```python
from build123d import *

# Parameters (mm, degrees)
BOSS_EXTRUDE1_DEPTH = 5.5
CUT_EXTRUDE1_DEPTH  = 3.5
SKETCH3_R           = 3
BOSS_EXTRUDE2_DEPTH = 3.5
SKETCH4_R           = 1.45
CUT_EXTRUDE2_DEPTH  = 5.5
SKETCH5_R           = 2.5
CUT_EXTRUDE3_DEPTH  = 2.6
CUT_EXTRUDE4_DEPTH  = 2
SKETCH7_W           = 3.5
SKETCH7_H           = 13.01
CUT_EXTRUDE5_DEPTH  = 1.55
SKETCH8_W           = 3.5
SKETCH8_H           = 12.6
CUT_EXTRUDE6_DEPTH  = 0.465


with BuildPart() as part:
    # Sketch1 → Boss-Extrude1 (new body)
    with BuildSketch(Plane.XY.offset(-5.5)):
        with BuildLine():
            Line((-30, -36), (30, -36))
            ThreePointArc((30, -36), (34.242640687, -34.242640687), (36, -30))
            Line((36, -30), (36, 30))
            ThreePointArc((36, 30), (34.242640687, 34.242640687), (30, 36))
            Line((30, 36), (-30, 36))
            ThreePointArc((-30, 36), (-34.242640687, 34.242640687), (-36, 30))
            Line((-36, 30), (-36, -30))
            ThreePointArc((-36, -30), (-34.242640687, -34.242640687), (-30, -36))
        make_face()
    extrude(amount=BOSS_EXTRUDE1_DEPTH)

    # Sketch2 → Cut-Extrude1 (cut)
    with BuildSketch(Plane.XY.offset(-3.5)):
        with BuildLine():
            Line((-30, -34), (30, -34))
            ThreePointArc((30, -34), (32.828427125, -32.828427125), (34, -30))
            Line((34, -30), (34, 30))
            ThreePointArc((34, 30), (32.828427125, 32.828427125), (30, 34))
            Line((30, 34), (-30, 34))
            ThreePointArc((-30, 34), (-32.828427125, 32.828427125), (-34, 30))
            Line((-34, 30), (-34, -30))
            ThreePointArc((-34, -30), (-32.828427125, -32.828427125), (-30, -34))
        make_face()
    extrude(amount=CUT_EXTRUDE1_DEPTH, mode=Mode.SUBTRACT)

    # Sketch3 → Boss-Extrude2 (add)
    with BuildSketch(Plane.XY.offset(-3.5)):
        with Locations((-30, 30)):
            Circle(SKETCH3_R)
        with Locations((30, 30)):
            Circle(SKETCH3_R)
        with Locations((-30, -30)):
            Circle(SKETCH3_R)
        with Locations((30, -30)):
            Circle(SKETCH3_R)
    extrude(amount=BOSS_EXTRUDE2_DEPTH)

    # Sketch4 → Cut-Extrude2 (cut)
    with BuildSketch(Plane.XY.offset(-5.5)):
        with Locations((-30, 30)):
            Circle(SKETCH4_R)
        with Locations((30, 30)):
            Circle(SKETCH4_R)
        with Locations((-30, -30)):
            Circle(SKETCH4_R)
        with Locations((30, -30)):
            Circle(SKETCH4_R)
    extrude(amount=CUT_EXTRUDE2_DEPTH, mode=Mode.SUBTRACT)

    # Sketch5 → Cut-Extrude3 (cut)
    with BuildSketch(Plane.XY.offset(-5.5)):
        with Locations((-30, 30)):
            Circle(SKETCH5_R)
        with Locations((30, 30)):
            Circle(SKETCH5_R)
        with Locations((-30, -30)):
            Circle(SKETCH5_R)
        with Locations((30, -30)):
            Circle(SKETCH5_R)
    extrude(amount=CUT_EXTRUDE3_DEPTH, mode=Mode.SUBTRACT)

    # Sketch6 → Cut-Extrude4 (cut)
    with BuildSketch(Plane.XY.offset(-5.5)):
        with BuildLine():
            Line((-16, -14), (-16, 14))
            ThreePointArc((-16, 14), (-15, 15), (-14, 14))
            Line((-14, 14), (-14, -14))
            ThreePointArc((-14, -14), (-15, -15), (-16, -14))
        make_face()
        with BuildLine():
            Line((-11, -14), (-11, 14))
            ThreePointArc((-11, 14), (-10, 15), (-9, 14))
            Line((-9, 14), (-9, -14))
            ThreePointArc((-9, -14), (-10, -15), (-11, -14))
        make_face()
        with BuildLine():
            Line((-6, -14), (-6, 14))
            ThreePointArc((-6, 14), (-5, 15), (-4, 14))
            Line((-4, 14), (-4, -14))
            ThreePointArc((-4, -14), (-5, -15), (-6, -14))
        make_face()
        with BuildLine():
            Line((-1, -14), (-1, 14))
            ThreePointArc((-1, 14), (0, 15), (1, 14))
            Line((1, 14), (1, -14))
            ThreePointArc((1, -14), (0, -15), (-1, -14))
        make_face()
        with BuildLine():
            Line((4, -14), (4, 14))
            ThreePointArc((4, 14), (5, 15), (6, 14))
            Line((6, 14), (6, -14))
            ThreePointArc((6, -14), (5, -15), (4, -14))
        make_face()
        with BuildLine():
            Line((9, -14), (9, 14))
            ThreePointArc((9, 14), (10, 15), (11, 14))
            Line((11, 14), (11, -14))
            ThreePointArc((11, -14), (10, -15), (9, -14))
        make_face()
        with BuildLine():
            Line((14, -14), (14, 14))
            ThreePointArc((14, 14), (15, 15), (16, 14))
            Line((16, 14), (16, -14))
            ThreePointArc((16, -14), (15, -15), (14, -14))
        make_face()
    extrude(amount=CUT_EXTRUDE4_DEPTH, mode=Mode.SUBTRACT)

    # Sketch7 → Cut-Extrude5 (cut)
    with BuildSketch(Plane.XY.offset(-1.55)):
        with Locations((35.25, -1.445)):
            Rectangle(SKETCH7_W, SKETCH7_H)
        with Locations((35.25, -20.495)):
            Rectangle(SKETCH7_W, SKETCH7_H)
    extrude(amount=CUT_EXTRUDE5_DEPTH, mode=Mode.SUBTRACT)

    # Sketch8 → Cut-Extrude6 (cut)
    with BuildSketch(Plane.XY.offset(-0.465)):
        with Locations((-35.25, -19)):
            Rectangle(SKETCH8_W, SKETCH8_H)
    extrude(amount=CUT_EXTRUDE6_DEPTH, mode=Mode.SUBTRACT)


solid = part.part
```
Read the model definition and answer for the solid it produces. Units are mm, in the model's axes. A direction names the side the tool comes from. Coordinates: 2 decimals unless noted, no trailing zeros. Write each loop counter-clockwise with the first axis right and the second up, starting at its lowest first coordinate (ties: lowest second). Pieces come first, ordered by that corner, then holes. Notation, with made-up numbers: (25, 65) -> (76, 65) arc R21 cw to (76, 92) -> close; hole circle Ø6 at (89, 24). An arc over 180 degrees is marked (long way). Answer as a JSON object with one key per item and string values.
Q1. A tool of negligible diameter and unlimited length cuts with its end or side. For faces 1 (the flat face through (-16, 0, -5)), 2 (the flat face through (32, -30, -2.9)), 3 (the cylindrical face through (27, 30, -2)), from which of +Z, -Z, +X, -X, +Y, -Y can it reach the whole face along a straight path? Write none if from no direction.
The answers:
{"face 1": "+Z, -Z", "face 2": "-Z", "face 3": "+Z"}
Q2. The part is cut by section C-C on z = -4.6. Give the number of separate pieces and of enclosed holes in the cut face, then the cut area to 3 significant figures.
The answers:
{"separate pieces": "1", "enclosed holes": "11", "area": "4,660 mm2"}
Q3. Determine the mould class of faces 4 (the cylindrical face through (-34.289, -34.196, -2.788)), 5 (the flat face through (35, -11, 0)), 6 (the flat face through (-6, 0, -5)) for opening direction Y: pulls with the +Y half, pulls with the -Y half, needs draft (parallel to the pull), parting line crosses it, or undercut.
The answers:
{"face 4": "pulls with the -Y half", "face 5": "needs draft", "face 6": "undercut"}
Q4. The part is cut by section B-B on y = 24. Give the vertices of the cut face in (x, z).
The answers:
{"outline": "(-36, -5.5) -> (36, -5.5) -> (36, 0) -> (34, 0) -> (34, -3.5) -> (-34, -3.5) -> (-34, 0) -> (-36, 0) -> close"}
Q5. The part is cut by section A-A on x = -5. Give the vertices of the cut face in (y, z), then the cut area to 3 significant figures.
The answers:
{"outline": "(-36, -5.5) -> (-15, -5.5) -> (-15, -3.5) -> (-34, -3.5) -> (-34, 0) -> (-36, 0) -> close; (15, -5.5) -> (36, -5.5) -> (36, 0) -> (34, 0) -> (34, -3.5) -> (15, -3.5) -> close", "area": "98.0 mm2"}
Q6. Consider line 1 (Y direction, x = 30, z = -2.05); line 2 (X direction, y = 32, z = -5.15); line 3 (Y direction, x = 10, z = -2.75). Determine where each line is inside the solid, lowest interval first. Write a range as [from, to].
The answers:
{"line 1": "y = [-36, -34], [-33, -31.45], [-28.55, -27], [27, 28.55], [31.45, 33], [34, 36]", "line 2": "x = [-35.66, -31.5], [-28.5, 28.5], [31.5, 35.66]", "line 3": "y = [-36, -34], [34, 36]"}
Q7. Flat-ended cylindrical pins translate along their axes: pin 1 Ø1.2 at (x, z) = (34.5, -0.5) entering from +Y; pin 2 Ø2.5 at (x, y) = (-30, 29) entering from -Z; pin 3 Ø1.5 at (x, y) = (12.5, -10.5) entering from +Z; pin 4 Ø2.5 at (x, y) = (30, -30) entering from +Z. Find the tip coordinate at first contact, or state that the pin passes through.
The answers:
{"pin 1": "stops at y = 34.56", "pin 2": "stops at z = -2.9", "pin 3": "stops at z = -3.5", "pin 4": "passes through"}
